from build123d import *

# Parameters (mm, degrees)
F0_W     = 250
F0_H     = 120
F1_DEPTH = 100
F2_R     = 10
F3_T     = -0.5
F4_R     = 3


with BuildPart() as f1:
    # F0 (on Top) → F1 (new body)
    with BuildSketch(Plane.XY):
        with Locations((125, 60)):
            Rectangle(F0_W, F0_H)
    extrude(amount=F1_DEPTH)

    # F2
    f2_edges = [f1.edges().sort_by_distance(p)[0] for p in [
        (0, 0, 50),
        (250, 0, 50),
        (250, 120, 50),
        (0, 120, 50),
    ]]
    fillet(f2_edges, radius=F2_R)

    # F3
    f3_openings = [f1.faces().sort_by_distance(p)[0] for p in [
        (125, 60, 100),
    ]]
    offset(amount=F3_T, openings=f3_openings)

    # F4
    f4_edges = [f1.edges().sort_by_distance(p)[0] for p in [
        (0.5, 60, 0.5),
        (3.282486, 3.282486, 0.5),
        (125, 0.5, 0.5),
        (246.717514, 3.282486, 0.5),
        (249.5, 60, 0.5),
        (246.717514, 116.717514, 0.5),
        (125, 119.5, 0.5),
        (3.282486, 116.717514, 0.5),
    ]]
    fillet(f4_edges, radius=F4_R)


solid = f1.part
Geometry check sheet. Reference: the model listing, model coordinates, mm. A direction names the side the tool comes from. Give positions to 0.01 mm unless a question says otherwise; leave off trailing zeros. Order: outer loops, then holes, each group sorted by start corner. A loop starts at its lowest first (then second) coordinate and runs counter-clockwise, first axis right, second up. Notation, with made-up numbers: M -26.5,1 L -17.5,1 A35 ccw -17.5,39 Z; hole C 24.5,46 d2. An arc over 180 degrees is marked long. Use a Markdown table: item, result.
Item 1: Material ranges on line 1 along Y through (x, z) = (44.5, 10.5); line 2 along X through (y, z) = (28, 74); line 3 along Z through (x, y) = (216.5, 34), recorded low to high.
Answers follow:
| item | result |
|---|---|
| line 1 | y = 0 to 0.5, 119.5 to 120 |
| line 2 | x = 0 to 0.5, 249.5 to 250 |
| line 3 | z = 0 to 0.5 |
Item 2: Tool access check on faces 1 (the cylindrical face through (2.85, 3.01, 50.7)), 2 (the flat face through (249.5, 59, 51)). Record the directions out of +Z, -Z, +X, -X, +Y, -Y that give a thin tool (end or side, any length) a straight path to the whole face; none if there is none.
Answers follow:
| item | result |
|---|---|
| face 1 | +Z, -Z, -X, -Y |
| face 2 | +Z |
Item 3: Depth check by flat-ended pin: P1, Ø12, axis at x = 118.5, y = 30, coming from the +Z side. Enter the tip coordinate at first touch or a pass-through.
Answers follow:
| item | result |
|---|---|
| P1 | stops at z = 0.5 |
Item 4: Section check B-B (x = 109). Record the cut outline in (y, z).
Answers follow:
| item | result |
|---|---|
| outline | M 0,0 L 120,0 L 120,100 L 119.5,100 L 119.5,3.5 A3 cw 116.5,0.5 L 3.5,0.5 A3 cw 0.5,3.5 L 0.5,100 L 0,100 Z |
Item 5: Draft check along X on faces 3 (the flat face through (123, 120, 49)), 4 (the cylindrical face through (246.99, 2.85, 50.7)), 5 (the cylindrical face through (3.209, 3.357, 52.426)). Enter one of: +X half, -X half, draft (parallel to the pull), parting line (faces both ways), or undercut.
Answers follow:
| item | result |
|---|---|
| face 3 | draft |
| face 4 | +X half |
| face 5 | undercut |
Item 6: Section check C-C (y = 47.5). Record the cut outline in (x, z).
Answers follow:
| item | result |
|---|---|
| outline | M 0,0 L 250,0 L 250,100 L 249.5,100 L 249.5,3.5 A3 cw 246.5,0.5 L 3.5,0.5 A3 cw 0.5,3.5 L 0.5,100 L 0,100 Z |
Item 7: Section check A-A (z = 42.5). Record the cut outline in (x, y), and give its area (3 significant figures).
Answers follow:
| item | result |
|---|---|
| outline | M 0,10 A10 ccw 10,0 L 240,0 A10 ccw 250,10 L 250,110 A10 ccw 240,120 L 10,120 A10 ccw 0,110 Z; hole M 0.5,10 A9.5 ccw 10,0.5 L 240,0.5 A9.5 ccw 249.5,10 L 249.5,110 A9.5 ccw 240,119.5 L 10,119.5 A9.5 ccw 0.5,110 Z |
| area | 361 mm2 |
